Can you work these out from the model? Positions are in its coordinate system, mm. A direction names the side the tool comes from. Give positions to 0.01 mm unless a question says otherwise; leave off trailing zeros. Order: outer loops, then holes, each group sorted by start corner. A loop starts at its lowest first (then second) coordinate and runs counter-clockwise, first axis right, second up. Notation, with made-up numbers: (50, 44) -> (59, 44) arc R13 cw to (59, 51) -> close; hole circle Ø4 at (89, -33.5). An arc over 180 degrees is marked (long way). Answer as a JSON object with one key per item and string values.
```python
from build123d import *

# Parameters (mm, degrees)
F2_R     = 5.5
F2_R_2   = 4
F3_DEPTH = 1
F2_R_3   = 2
F4_DEPTH = 6
F5_R     = 0.8


with BuildPart() as f1:
    # F0 (on Front) → F1 (revolve)
    with BuildSketch(Plane.XZ):
        with BuildLine():
            Line((-11, 0), (0, 0))
            Line((0, 0), (0, 1.5))
            ThreePointArc((0, 1.5), (-4.154055, 1.744273), (-8.171573, 2.828427))
            Line((-8.171573, 2.828427), (-11, 0))
        make_face()
    revolve(axis=Axis((0, 0, 0.75), (0, 0, 1)))

    # F2 (on face) → F3 (join)
    with BuildSketch(Plane(origin=(0, 0, 0), x_dir=(1, 0, 0), z_dir=(0, 0, -1))):
        Circle(F2_R)
        Circle(F2_R_2, mode=Mode.SUBTRACT)
    extrude(amount=F3_DEPTH)

    # F2 (on face) → F4 (join)
    with BuildSketch(Plane(origin=(0, 0, 0), x_dir=(1, 0, 0), z_dir=(0, 0, -1))):
        Circle(F2_R_2)
        Circle(F2_R_3, mode=Mode.SUBTRACT)
    extrude(amount=F4_DEPTH)

    # F5
    f5_edges = [f1.edges().sort_by_distance(p)[0] for p in [
        (-2, 0, -6),
    ]]
    fillet(f5_edges, radius=F5_R)


solid = f1.part
```
1. Please list where these lines run through material, in increasing order: L1, parallel to Y at x = 0, z = -3.25; L2, parallel to Z at x = -9.5, y = 0.
Worked answers:
{"L1": "-4 to -2, 2 to 4", "L2": "0 to 1.5"}
2. For faces 4 (the face through (0, 0, 0)), 5 (the face through (1, -3, -6)), which set-ups out of +Z, -Z, +X, -X, +Y, -Y let a thin tool reach every point of the face, with its end or its side?
Worked answers:
{"face 4": "-Z", "face 5": "-Z, +X, -X, +Y, -Y"}
3. Will these pins go through, and if not, where does the flat tip stop? pin 1 Ø12 at (x, y) = (1.5, 8.5) entering from -Z; pin 2 Ø1.5 at (x, y) = (0, 5.5) entering from +Z; pin 3 Ø2 at (x, y) = (0, 0.5) entering from -Z; pin 4 Ø2.5 at (x, y) = (0, 0) entering from +Z.
Worked answers:
{"pin 1": "z = -6", "pin 2": "z = 2.2", "pin 3": "z = 0", "pin 4": "z = 1.5"}
4. If we section it at A-A on z = -4: Please give me the cut outline in (x, y), then the cut area to 3 significant figures.
Worked answers:
{"outline": "circle Ø8 at (0, 0); hole circle Ø4 at (0, 0)", "area": "37.7 mm²"}
5. If we mould it in two halves opening along Y, with no side actions, what happens to faces 1 (the face through (0, 2, -3)), 2 (the face through (-7.963, -2.508, 2.651)), 3 (the face through (3, -5, 0))? For each: +Y half, -Y half, draft (parallel to the pull), parting line (faces both ways), or undercut.
Worked answers:
{"face 1": "undercut", "face 2": "parting line", "face 3": "draft"}
